```python
from build123d import *

# Parameters (mm, degrees)
F1_DEPTH = 6.5
F2_R     = 1.45
F3_DEPTH = 25
F4_R     = 1.45
F5_DEPTH = 25


with BuildPart() as f1:
    # F0 (on Front) → F1 (new body)
    with BuildSketch(Plane.XZ):
        with BuildLine():
            ThreePointArc((-5.15, 0), (0, 5.15), (5.15, 0))
            Line((5.15, 0), (6.15, 0))
            Line((6.15, 0), (10.362235, -4.212235))
            Line((10.362235, -4.212235), (12.483555, -2.090915))
            Line((12.483555, -2.090915), (3.280338, 7.112302))
            Line((3.280338, 7.112302), (-3.280338, 7.112302))
            Line((-3.280338, 7.112302), (-12.483555, -2.090915))
            Line((-12.483555, -2.090915), (-10.362235, -4.212235))
            Line((-10.362235, -4.212235), (-6.15, 0))
            Line((-6.15, 0), (-5.15, 0))
        make_face()
    extrude(amount=F1_DEPTH)

    # F2 (on face) → F3 (cut)
    with BuildSketch(Plane(origin=(-5.19632, 0, 5.19632), x_dir=(0, -1, 0), z_dir=(-0.707107, 0, 0.707107))):
        with Locations((3.25, -7.327207)):
            Circle(F2_R)
    extrude(amount=-F3_DEPTH, mode=Mode.SUBTRACT)

    # F4 (on face) → F5 (cut)
    with BuildSketch(Plane(origin=(5.19632, 0, 5.19632), x_dir=(0, 1, 0), z_dir=(0.707107, 0, 0.707107))):
        with Locations((-3.25, -7.327207)):
            Circle(F4_R)
    extrude(amount=-F5_DEPTH, mode=Mode.SUBTRACT)


solid = f1.part
```
Design review of the part built by this model. Coordinates are the model's own, in mm. A direction names the side the tool comes from. Coordinates: 2 decimals unless noted, no trailing zeros. Order: outer loops, then holes, each group sorted by start corner. A loop starts at its lowest first (then second) coordinate and runs counter-clockwise, first axis right, second up. Notation, with made-up numbers: M 0.25,24 L 27.25,24 A10 ccw 27.25,33 Z; hole C 55,52 d7. An arc over 180 degrees is marked long. Answer as a JSON object with one key per item and string values. Group by question number.
1) Tool access review of faces 4 (the flat face through (7.76, -1.76, -1.61)), 5 (the flat face through (0, -3, 7.112)): name each direction out of +Z, -Z, +X, -X, +Y, -Y from which nothing blocks a thin tool from reaching the whole face with its end or side.
2) Add section C-C, the plane x = 0. Write out the cut boundary in (y, z), then the cut area to 3 significant figures.
3) For pin 1 (4 mm diameter, centred on x = -3.5, z = 2, fed in from -Y); pin 2 (0.5 mm diameter, centred on x = 5.5, y = -2.5, fed in from -Z); pin 3 (1 mm diameter, centred on y = -2.5, z = -0.5, fed in from +X), all flat-tipped, find the tip position at first contact; note any pin that passes through.
4) Add section B-B, the plane y = -3.25. Write out the cut boundary in (x, z).
5) Add section A-A, the plane y = -1.5. Write out the cut boundary in (x, z), then the cut area to 3 significant figures.
6) Add section D-D, the plane z = 6.75. Write out the cut boundary in (x, y).
7) Mouldability with a two-part tool opening along X and no side actions: class faces 1 (the flat face through (-8.75, -1.76, -2.6)), 2 (the flat face through (11.408, -3.204, -3.166)), 3 (the flat face through (-1, 0, 5.3)) as pulls with the +X half, pulls with the -X half, needs draft (parallel to the pull), parting line crosses it, or undercut.
8) Wall thickness on L1, parallel to Z at x = 0, y = -4.25; L2, parallel to X at y = -1.75, z = -3; L3, parallel to X at y = -2.75, z = 4.5: over which ranges is each line inside the solid? List them lowest first.
Computed values:
{
 "1": {"face 4": "-Z, +Y, -Y", "face 5": "+Z, +X, -X, +Y, -Y"},
 "2": {"outline": "M -6.5,5.15 L 0,5.15 L 0,7.11 L -6.5,7.11 Z", "area": "12.8 mm^2"},
 "3": {"pin 1": "stops at y = -6.5", "pin 2": "stops at z = 0", "pin 3": "stops at x = 11.39"},
 "4": {"outline": "M -12.48,-2.09 L -10.36,-4.21 L -9.28,-3.13 L -11.4,-1.01 Z; M -9.35,1.04 L -7.23,-1.08 L -6.15,0 L -5.15,0 A5.15 cw 5.15,0 L 6.15,0 L 7.23,-1.08 L 9.35,1.04 L 3.28,7.11 L -3.28,7.11 Z; M 9.28,-3.13 L 10.36,-4.21 L 12.48,-2.09 L 11.4,-1.01 Z"},
 "5": {"outline": "M -12.48,-2.09 L -10.36,-4.21 L -6.15,0 L -5.15,0 A5.15 cw 5.15,0 L 6.15,0 L 10.36,-4.21 L 12.48,-2.09 L 3.28,7.11 L -3.28,7.11 Z", "area": "82.3 mm^2"},
 "6": {"outline": "M -3.64,-6.5 L 3.64,-6.5 L 3.64,0 L -3.64,0 Z"},
 "7": {"face 1": "undercut", "face 2": "pulls with the +X half", "face 3": "needs draft"},
 "8": {"L1": "z = 5.15 to 7.11", "L2": "x = -11.57 to -9.15, 9.15 to 11.57", "L3": "x = -5.89 to -2.5, 2.5 to 5.89"}
}
